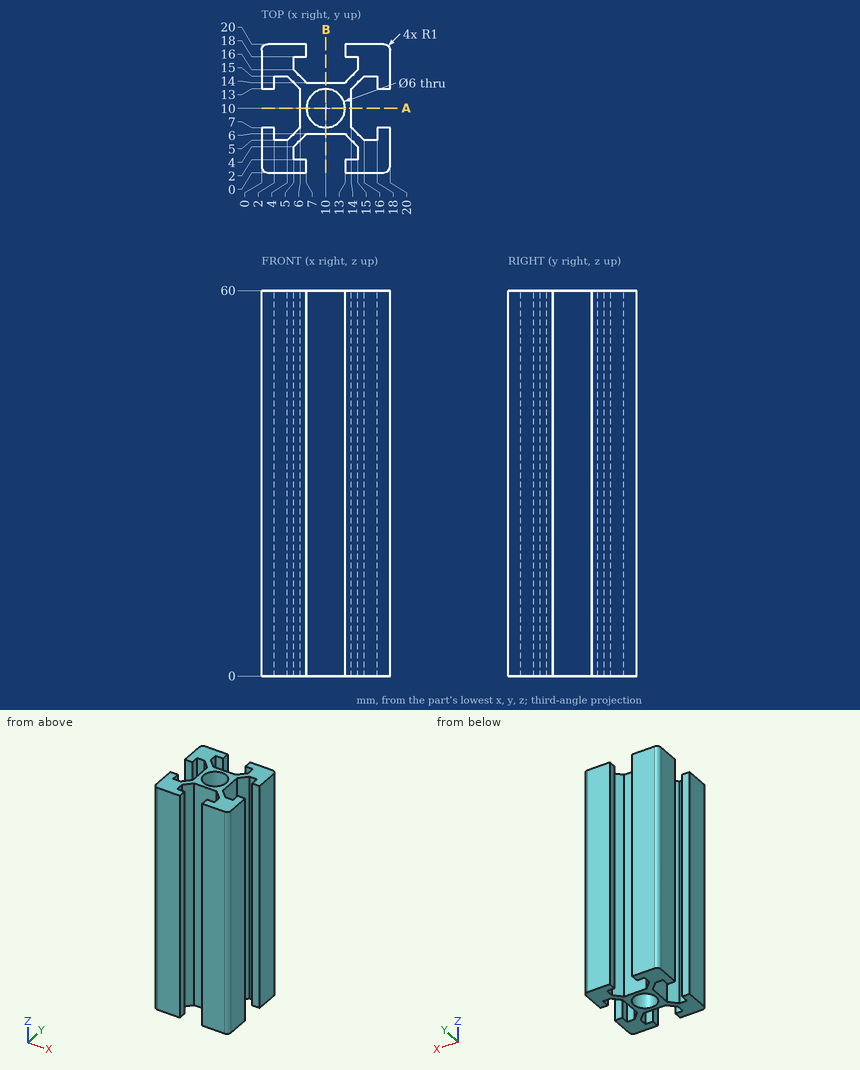
Verification items for this drawing (mm, ordinates from the low corner). Coordinates: 2 decimals unless noted, no trailing zeros. Loops run counter-clockwise (first coordinate to the right, second up) from the corner with the lowest first, then second, coordinate; pieces in that order, holes last.
Item 1: Sectioned sample at A-A, the plane y = 10. Record the boundary of the cut face in (x, z), then the cut area to 3 significant figures.
Item 2: Thickness scan on line 1 (Y direction, x = 10, z = 40.5); line 2 (X direction, y = 13.5, z = 53.5); line 3 (Y direction, x = 16, z = 35). Record the ranges inside material, lowest first.
Item 3: Go/stop test with flat-tipped pins: pin 1 Ø1.5 at (x, z) = (10, 21) entering from +Y; pin 2 Ø3 at (y, z) = (9, 35) entering from -X. Record where each tip stops, or that it passes through.
Check result:
1. outline: (6, 0) - (7, 0) - (7, 60) - (6, 60) - close; (13, 0) - (14, 0) - (14, 60) - (13, 60) - close
1. area: 120 mm2
2. line 1: y = 6 to 7, 13 to 14
2. line 2: x = 0 to 2, 5.5 to 14.5, 18 to 20
2. line 3: y = 0 to 5, 15 to 20
3. pin 1: stops at y = 14
3. pin 2: stops at x = 6
